For this review, take the finished solid that the model builds, in its own axes (mm). A direction names the side the tool comes from. Round coordinates to 2 decimals unless told otherwise and drop trailing zeros. Order: outer loops, then holes, each group sorted by start corner. A loop starts at its lowest first (then second) coordinate and runs counter-clockwise, first axis right, second up. Notation, with made-up numbers: (47, 67) -> (58, 67) arc R10 ccw to (58, 78) -> close; hole circle Ø3 at (-32.5, -27). An arc over 180 degrees is marked (long way). Answer in a Markdown table with one row per item.
Autodesk Inventor part; units mm, degrees
ref_plane "YZ Plane" through (0, 0, 0) normal (1, 0, 0) x (0, 1, 0)
ref_plane "XZ Plane" through (0, 0, 0) normal (0, 1, 0) x (-1, 0, 0)
ref_plane "XY Plane" through (0, 0, 0) normal (0, 0, 1) x (1, 0, 0)
sketch "Sketch1" plane through (0, 0, 0) normal (0, 1, 0) x (-1, 0, 0)
  line L0 (-70, 35) -> (70, 35)
  line L1 (75, 30) -> (75, -30)
  line L2 (70, -35) -> (-70, -35)
  line L3 (-75, -30) -> (-75, 30)
  line L4 (-75, 35) -> (75, -35) construction
  line L5 (75, 35) -> (-75, -35) construction
  arc A0 (75, 30) -> (70, 35) centre (70, 30) ccw
  arc A1 (70, -35) -> (75, -30) centre (70, -30) ccw
  arc A2 (-70, 35) -> (-75, 30) centre (-70, 30) ccw
  arc A3 (-75, -30) -> (-70, -35) centre (-70, -30) ccw
  line L6 (-72, 37) -> (72, 37)
  line L7 (77, 32) -> (77, -32)
  line L8 (72, -37) -> (-72, -37)
  line L9 (-77, -32) -> (-77, 32)
  line L10 (-77, 37) -> (77, -37) construction
  line L11 (77, 37) -> (-77, -37) construction
  arc A4 (77, 32) -> (72, 37) centre (72, 32) ccw
  arc A5 (72, -37) -> (77, -32) centre (72, -32) ccw
  arc A6 (-77, -32) -> (-72, -37) centre (-72, -32) ccw
  arc A7 (-72, 37) -> (-77, 32) centre (-72, 32) ccw
  line L12 (74, 39) -> (-74, 39)
  line L13 (-79, 34) -> (-79, -34)
  line L14 (-74, -39) -> (74, -39)
  line L15 (79, -34) -> (79, 34)
  line L16 (79, 39) -> (-79, -39) construction
  line L17 (-79, 39) -> (79, -39) construction
  arc A8 (79, 34) -> (74, 39) centre (74, 34) ccw
  arc A9 (-74, 39) -> (-79, 34) centre (-74, 34) ccw
  arc A10 (-79, -34) -> (-74, -39) centre (-74, -34) ccw
  arc A11 (74, -39) -> (79, -34) centre (74, -34) ccw
  point P0 (0, 0)
  point P1 (0, 0)
  point P2 (0, 0)
  dimension "d0" = 150
  dimension "d1" = 70
  dimension "d2" = 5
  dimension "d3" = 2
  dimension "d4" = 2
  dimension "d5" = 5
  dimension "d6" = 4
  dimension "d7" = 4
  dimension "d8" = 5
extrude "Extrusion1" add sketch "Sketch1" along normal blind 2 contours A8 L15 A11 L14 A10 L13 A9 L12
properties part number "Box2_spacer"
Q1. Take a section at A-A, the plane x = -42.5. Write out the cut boundary in (y, z), then the cut area to 3 significant figures.
Answer key:
| item | result |
|---|---|
| outline | (0, -39) -> (2, -39) -> (2, -37) -> (0, -37) -> close; (0, 37) -> (2, 37) -> (2, 39) -> (0, 39) -> close |
| area | 8.00 mm^2 |
Q2. Take a section at B-B, the plane z = 0. Write out the cut boundary in (x, y), then the cut area to 3 significant figures.
Answer key:
| item | result |
|---|---|
| outline | (-79, 0) -> (-77, 0) -> (-77, 2) -> (-79, 2) -> close; (77, 0) -> (79, 0) -> (79, 2) -> (77, 2) -> close |
| area | 8.00 mm^2 |
Q3. The part is to be moulded in two halves that separate along Z. For faces 1 (the face through (-76, 1, -35)), 2 (the face through (77, 1, -38)), 3 (the face through (-77, 1, 38)), say which applies: +Z half, -Z half, draft (parallel to the pull), parting line (faces both ways), or undercut.
Answer key:
| item | result |
|---|---|
| face 1 | undercut |
| face 2 | -Z half |
| face 3 | +Z half |
Q4. Take a section at C-C, the plane y = 0.6. Write out the cut boundary in (x, z), then the cut area to 3 significant figures.
Answer key:
| item | result |
|---|---|
| outline | (-79, -34) arc R5 ccw to (-74, -39) -> (74, -39) arc R5 ccw to (79, -34) -> (79, 34) arc R5 ccw to (74, 39) -> (-74, 39) arc R5 ccw to (-79, 34) -> close; hole (-77, -32) arc R5 ccw to (-72, -37) -> (72, -37) arc R5 ccw to (77, -32) -> (77, 32) arc R5 ccw to (72, 37) -> (-72, 37) arc R5 ccw to (-77, 32) -> close |
| area | 928 mm^2 |
Q5. Tool access review of faces 4 (the face through (76, 1, 35)), 5 (the face through (78, 1, 37)): name each direction out of +Z, -Z, +X, -X, +Y, -Y from which nothing blocks a thin tool from reaching the whole face with its end or side.
Answer key:
| item | result |
|---|---|
| face 4 | +Y, -Y |
| face 5 | +Z, +X, +Y, -Y |
Q6. To check wall thickness, follow probe 1 along Z at (x, y) = (-66, 0.6); probe 2 along X at (y, z) = (0.1, 7). State the ranges of each line that lie inside material, in increasing order.
Answer key:
| item | result |
|---|---|
| probe 1 | z = -39 to -37, 37 to 39 |
| probe 2 | x = -79 to -77, 77 to 79 |
